Model file for the job. Use its own axes, mm. Coordinates: 2 decimals unless noted, no trailing zeros. Order: outer loops, then holes, each group sorted by start corner. A loop starts at its lowest first (then second) coordinate and runs counter-clockwise, first axis right, second up. Notation, with made-up numbers: (-36.75, 24.25) -> (16.25, 24.25) arc R28 ccw to (16.25, 46.25) -> close; hole circle Ø3 at (80.25, 33.25). An arc over 180 degrees is marked (long way). Use CSV: the item, a comma, the result in double quotes. Start each with the question number.
(1) Probe L1, parallel to X at y = 0.2, z = 0.5; L2, parallel to Z at x = -59.5, y = 0.2; L3, parallel to X at y = 1.2, z = 1.45. List the from-to ranges inside material, lowest first.
(2) Pin check, flat tips, straight feed: pin 1 Ø1 at (x, y) = (-38, 0.5) entering from -Z; pin 2 Ø2.5 at (x, y) = (-24.5, 0.5) entering from +Z; pin 3 Ø1 at (y, z) = (1, 2.5) entering from -X. Stop position of each tip, or through.
(3) Pull direction X, two halves, no side cores. Call faces 1 (the cylindrical face through (51.617, -0.67, 1.539)), 2 (the flat face through (50, 0, 2.8)), 3 (the cylindrical face through (-48.383, -0.67, 1.539)): pulls with the +X half, pulls with the -X half, needs draft (parallel to the pull), parting line crosses it, or undercut.
(4) Cut at B-B on z = 1.3. Write the cut outline in (x, y).
(5) Cut at A-A on x = -50. Write the cut outline in (y, z), plus the area to 3 significant figures.
```python
from build123d import *

# Parameters (mm, degrees)
SKICA2_W                = 150
SKICA2_H                = 4.6
SKICA2_W_2              = 18
SKICA2_H_2              = 1
P_IDAT_VYSUNUT_M2_DEPTH = 0.8
SKICA3_R                = 1.75
P_IDAT_VYSUNUT_M3_DEPTH = 2
ZAOBLIT1_R              = 0.5
SKICA4_W                = 0.6
SKICA4_H                = 1
P_IDAT_VYSUNUT_M4_DEPTH = 0.8
ZKOSEN_1_SIZE           = 0.4
ZKOSEN_1_SIZE2          = 0.145588094
ZKOSEN_1_PART_2_SIZE    = 0.4
ZKOSEN_1_PART_2_SIZE2   = 0.145588094
ZKOSEN_1_PART_3_SIZE    = 0.4
ZKOSEN_1_PART_3_SIZE2   = 0.145588094
ZKOSEN_1_PART_4_SIZE    = 0.4
ZKOSEN_1_PART_4_SIZE2   = 0.145588094


with BuildPart() as part:
    # Skica2 → Přidat vysunutím2 (new body)
    with BuildSketch(Plane.XY):
        Rectangle(SKICA2_W, SKICA2_H)
        with Locations((-5, 0)):
            Rectangle(SKICA2_W_2, SKICA2_H_2, mode=Mode.SUBTRACT)
    extrude(amount=P_IDAT_VYSUNUT_M2_DEPTH)

    # Skica3 → Přidat vysunutím3 (add)
    with BuildSketch(Plane.XY.offset(0.8)):
        with Locations((-50, 0)):
            Circle(SKICA3_R)
        with Locations((50, 0)):
            Circle(SKICA3_R)
    extrude(amount=P_IDAT_VYSUNUT_M3_DEPTH)

    # Zaoblit1
    zaoblit1_edges = [part.edges().sort_by_distance(p)[0] for p in [
        (-51.75, 0, 2.8),
        (48.25, 0, 2.8),
    ]]
    fillet(zaoblit1_edges, radius=ZAOBLIT1_R)

    # Skica4 → Přidat vysunutím4 (add)
    with BuildSketch(Plane(origin=(0, 0, 0), x_dir=(-1, 0, 0), z_dir=(0, 0, -1))):
        with Locations((1.9, 0)):
            Rectangle(SKICA4_W, SKICA4_H)
        with Locations((8.1, 0)):
            Rectangle(SKICA4_W, SKICA4_H)
    extrude(amount=-P_IDAT_VYSUNUT_M4_DEPTH)

    # Zkosení1
    zkosen_1_edges = [part.edges().sort_by_distance(p)[0] for p in [
        (-1.6, 0, 0),
    ]]
    zkosen_1_side = [part.faces().sort_by_distance(p)[0] for p in [
        (-1.6, 0, 0.4),
    ]]
    chamfer(zkosen_1_edges, length=ZKOSEN_1_SIZE, length2=ZKOSEN_1_SIZE2, reference=zkosen_1_side[0])

    # Zkosení1 part 2
    zkosen_1_part_2_edges = [part.edges().sort_by_distance(p)[0] for p in [
        (-2.2, 0, 0),
    ]]
    zkosen_1_part_2_side = [part.faces().sort_by_distance(p)[0] for p in [
        (-2.2, 0, 0.4),
    ]]
    chamfer(zkosen_1_part_2_edges, length=ZKOSEN_1_PART_2_SIZE, length2=ZKOSEN_1_PART_2_SIZE2, reference=zkosen_1_part_2_side[0])

    # Zkosení1 part 3
    zkosen_1_part_3_edges = [part.edges().sort_by_distance(p)[0] for p in [
        (-8.4, 0, 0),
    ]]
    zkosen_1_part_3_side = [part.faces().sort_by_distance(p)[0] for p in [
        (-8.4, 0, 0.4),
    ]]
    chamfer(zkosen_1_part_3_edges, length=ZKOSEN_1_PART_3_SIZE, length2=ZKOSEN_1_PART_3_SIZE2, reference=zkosen_1_part_3_side[0])

    # Zkosení1 part 4
    zkosen_1_part_4_edges = [part.edges().sort_by_distance(p)[0] for p in [
        (-7.8, 0, 0),
    ]]
    zkosen_1_part_4_side = [part.faces().sort_by_distance(p)[0] for p in [
        (-7.8, 0, 0.4),
    ]]
    chamfer(zkosen_1_part_4_edges, length=ZKOSEN_1_PART_4_SIZE, length2=ZKOSEN_1_PART_4_SIZE2, reference=zkosen_1_part_4_side[0])


solid = part.part
```
Outcome:
1,L1,"-75 to -14, -8.4 to -7.8, -2.2 to -1.6, 4 to 75"
1,L2,"0 to 0.8"
1,L3,"-51.27 to -48.73, 48.73 to 51.27"
2,pin 1,"z = 0"
2,pin 2,"z = 0.8"
2,pin 3,"x = -51.67"
3,face 1,"undercut"
3,face 2,"needs draft"
3,face 3,"undercut"
4,outline,"circle Ø3.5 at (-50, 0); circle Ø3.5 at (50, 0)"
5,outline,"(-2.3, 0) -> (2.3, 0) -> (2.3, 0.8) -> (1.75, 0.8) -> (1.75, 2.3) arc R0.5 ccw to (1.25, 2.8) -> (-1.25, 2.8) arc R0.5 ccw to (-1.75, 2.3) -> (-1.75, 0.8) -> (-2.3, 0.8) -> close"
5,area,"10.6 mm2"
